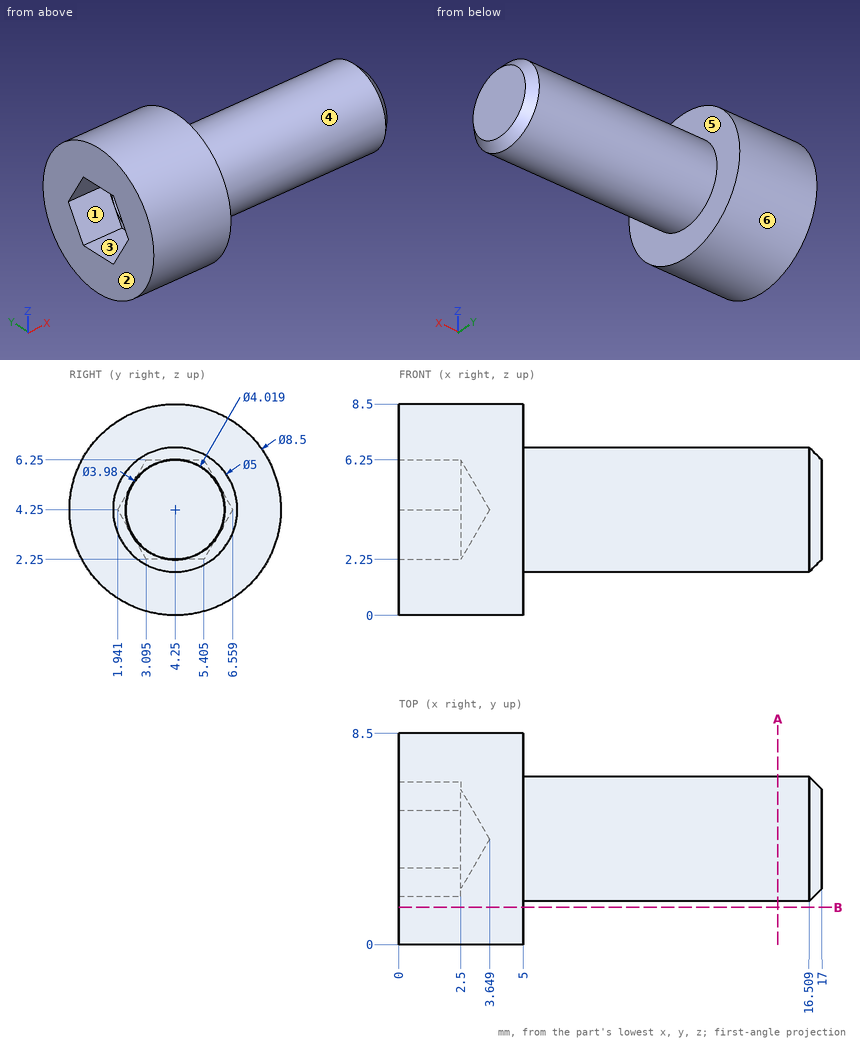
Print and shaded views of the part. All mm, measured from the part's lowest x, y and z. A direction names the side the tool comes from. Coordinates: 2 decimals unless noted, no trailing zeros. Order: outer loops, then holes, each group sorted by start corner. A loop starts at its lowest first (then second) coordinate and runs counter-clockwise, first axis right, second up.
Item 1: Drill centre lines: L1, parallel to X at y = 7.25, z = 3.5; L2, parallel to Z at x = 1.5, y = 4.5; L3, parallel to Y at x = 2.25, z = 5 (1 decimal). Where is each one in solid material? Low to high.
Filled in:
L1: x = 0 to 5
L2: z = 0.01 to 2.25, 6.25 to 8.49
L3: y = 0.1 to 2.4, 6.1 to 8.4
Item 2: Saw through at A-A on x = 15.25. List the corners of the cut face in (y, z).
Filled in:
outline: circle Ø5 at (4.25, 4.25)
Item 3: Saw through at B-B on y = 1.5. List the corners of the cut face in (x, z).
Filled in:
outline: (0, 1.01) - (5, 1.01) - (5, 7.49) - (0, 7.49) - close
Item 4: Tool access for the marked faces 5 and 6: list every direction of +Z, -Z, +X, -X, +Y, -Y with a clear straight run to the whole face (end or side of a thin tool).
Filled in:
face 5: +X
face 6: +X, -X
Item 5: Drop flat-ended pins along their axis: pin 1 Ø3 at (x, z) = (5, 1.5) entering from -Y; pin 2 Ø1.5 at (x, z) = (9.5, 1.5) entering from -Y; pin 3 Ø2 at (x, y) = (8, 6) entering from +Z (1 decimal). Give the stop position or say it passes through.
Filled in:
pin 1: stops at y = 0.19
pin 2: stops at y = 2.75
pin 3: stops at z = 6.6
Item 6: Mould opens along Y. For the marked faces 1, 2, 3 and 4 say: released by +Y, released by -Y, zero draft, split by the parting line, or undercut.
Filled in:
face 1: undercut
face 2: zero draft
face 3: undercut
face 4: split by the parting line
